from build123d import *

# Parameters (mm, degrees)
BOSS_EXTRUDE1_DEPTH = 4
FILLET1_R           = 3
SKETCH3_R           = 2.6
CUT_EXTRUDE1_DEPTH  = 4
SKETCH4_R           = 1.5
CUT_EXTRUDE2_DEPTH  = 4
SKETCH5_W           = 15
SKETCH5_H           = 20
BOSS_EXTRUDE2_DEPTH = 4
BOSS_EXTRUDE3_DEPTH = 4
SKETCH7_R           = 1.5
CUT_EXTRUDE3_DEPTH  = 4
BOSS_EXTRUDE4_DEPTH = 4
SKETCH10_R          = 11.5
CUT_EXTRUDE4_DEPTH  = 4
SKETCH14_R          = 1.5
CUT_EXTRUDE5_DEPTH  = 4
FILLET2_R           = 3
SKETCH17_W          = 41.796836064
SKETCH17_H          = 42.2
CUT_EXTRUDE6_DEPTH  = 10
FILLET3_R           = 3


with BuildPart() as part:
    # Sketch1 → Boss-Extrude1 (new body)
    with BuildSketch(Plane.XY):
        Polygon((39, 10), (39, 30), (-1, 30), (-9, 10), (-39, 10), (-39, -10), (-9, -10), (-1, -30), (39, -30), (39, -10), align=None)
    extrude(amount=BOSS_EXTRUDE1_DEPTH)

    # Fillet1
    fillet1_edges = [part.edges().sort_by_distance(p)[0] for p in [
        (39, -30, 2),
        (-1, -30, 2),
        (-9, -10, 2),
        (-39, -10, 2),
        (-39, 10, 2),
        (-9, 10, 2),
        (-1, 30, 2),
        (39, 30, 2),
    ]]
    fillet(fillet1_edges, radius=FILLET1_R)

    # Sketch3 → Cut-Extrude1 (cut)
    with BuildSketch(Plane.XY.offset(4)):
        with Locations((33, 20)):
            Circle(SKETCH3_R)
        with Locations((1.6, 20)):
            Circle(SKETCH3_R)
        with Locations((33, -20)):
            Circle(SKETCH3_R)
        with Locations((1.6, -20)):
            Circle(SKETCH3_R)
        with Locations((1.6, 0)):
            Circle(SKETCH3_R)
    extrude(amount=-CUT_EXTRUDE1_DEPTH, mode=Mode.SUBTRACT)

    # Sketch4 → Cut-Extrude2 (cut)
    with BuildSketch(Plane.XY.offset(4)):
        with Locations((-32, 0)):
            Circle(SKETCH4_R)
        with Locations((-25, 0)):
            Circle(SKETCH4_R)
        with Locations((-18, 0)):
            Circle(SKETCH4_R)
        with Locations((-11, 0)):
            Circle(SKETCH4_R)
        with Locations((32, 0)):
            Circle(SKETCH4_R)
        with Locations((25, 0)):
            Circle(SKETCH4_R)
        with Locations((18, 0)):
            Circle(SKETCH4_R)
    extrude(amount=-CUT_EXTRUDE2_DEPTH, mode=Mode.SUBTRACT)

    # Sketch5 → Boss-Extrude2 (add)
    with BuildSketch(Plane.XY.offset(4)):
        with Locations((46.5, 0)):
            Rectangle(SKETCH5_W, SKETCH5_H)
    extrude(amount=-BOSS_EXTRUDE2_DEPTH)

    # Sketch6 → Boss-Extrude3 (add)
    with BuildSketch(Plane.XY.offset(4)):
        Polygon((39, 10), (54, 10), (39, 27), align=None)
        Polygon((54, -10), (39, -10), (39, -27), align=None)
    extrude(amount=-BOSS_EXTRUDE3_DEPTH)

    # Sketch7 → Cut-Extrude3 (cut)
    with BuildSketch(Plane.XY.offset(4)):
        with Locations((46.5, 0)):
            Circle(SKETCH7_R)
    extrude(amount=-CUT_EXTRUDE3_DEPTH, mode=Mode.SUBTRACT)

    # Sketch8 → Boss-Extrude4 (add)
    with BuildSketch(Plane.XY.offset(4)):
        Polygon((54, -10), (54, -21.1), (96.2, -21.1), (96.2, 21.1), (54, 21.1), (54, 10), align=None)
        Polygon((44.205882353, 21.1), (54, 10), (54, 21.1), align=None)
        Polygon((44.205882353, -21.1), (54, -21.1), (54, -10), align=None)
    extrude(amount=-BOSS_EXTRUDE4_DEPTH)

    # Sketch10 → Cut-Extrude4 (cut)
    with BuildSketch(Plane.XY.offset(4)):
        with Locations((74.8, 0)):
            Circle(SKETCH10_R)
    extrude(amount=-CUT_EXTRUDE4_DEPTH, mode=Mode.SUBTRACT)

    # Sketch14 → Cut-Extrude5 (cut)
    with BuildSketch(Plane.XY.offset(4)):
        with Locations((90.674547238, 15.874547238)):
            Circle(SKETCH14_R)
        with Locations((58.925452762, -15.874547238)):
            Circle(SKETCH14_R)
        with Locations((58.925452762, 15.874547238)):
            Circle(SKETCH14_R)
        with Locations((90.674547238, -15.874547238)):
            Circle(SKETCH14_R)
    extrude(amount=-CUT_EXTRUDE5_DEPTH, mode=Mode.SUBTRACT)

    # Fillet2
    fillet2_edges = [part.edges().sort_by_distance(p)[0] for p in [
        (96.2, -21.1, 2),
        (44.205882353, -21.1, 2),
        (44.205882353, 21.1, 2),
        (96.2, 21.1, 2),
        (39, 27, 2),
    ]]
    fillet(fillet2_edges, radius=FILLET2_R)

    # Sketch17 → Cut-Extrude6 (cut)
    with BuildSketch(Plane.XY.offset(4)):
        with Locations((75.301581968, 0)):
            Rectangle(SKETCH17_W, SKETCH17_H)
    extrude(amount=-CUT_EXTRUDE6_DEPTH, mode=Mode.SUBTRACT)

    # Fillet3
    fillet3_edges = [part.edges().sort_by_distance(p)[0] for p in [
        (54.403163936, -21.1, 2),
        (54.403163936, 21.1, 2),
    ]]
    fillet(fillet3_edges, radius=FILLET3_R)


solid = part.part
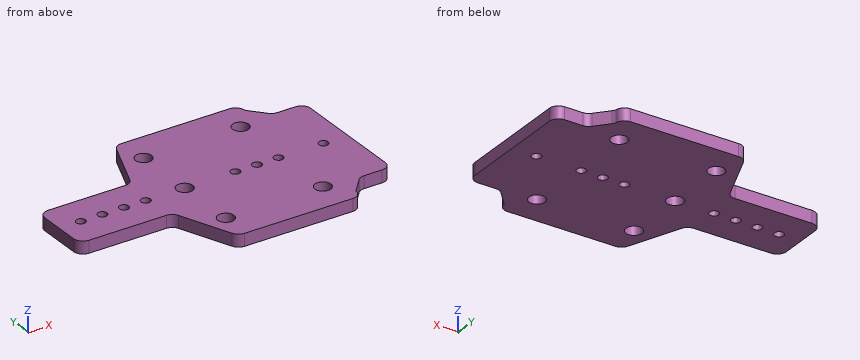
Design review of the part built by this model. Coordinates are the model's own, in mm. Coordinates: 2 decimals unless noted, no trailing zeros. Order: outer loops, then holes, each group sorted by start corner. A loop starts at its lowest first (then second) coordinate and runs counter-clockwise, first axis right, second up.
Item 1: For pin 1 Ø2.5 at (x, y) = (46.5, 0) entering from -Z; pin 2 Ø1.5 at (y, z) = (-12.5, 1) entering from -X; pin 3 Ø2 at (x, z) = (49, 1.5) entering from +Y; pin 4 Ø2 at (x, z) = (-19.5, 3) entering from +Y, all flat-tipped, find the tip position at first contact; note any pin that passes through.
Item 2: For line 1 (Y direction, x = 1.6, z = 1.3); line 2 (Y direction, x = 33, z = 0.9); line 3 (X direction, y = 19.5, z = 2.15), list the stretches that pass through material, from the lowest coordinate up.
Item 3: Take a section at C-C, the plane x = 46.5. Write out the cut boundary in (y, z).
Item 4: Take a section at B-B, the plane y = 0. Count the separate pieces of the cut face and the enclosed holes in it, then the cut area to 3 significant figures.
Item 5: Take a section at A-A, the plane x = 18. Write out the cut boundary in (y, z), then the cut area to 3 significant figures.
The answers:
1. pin 1: passes through
1. pin 2: stops at x = -8.3
1. pin 3: stops at y = 21.1
1. pin 4: stops at y = 10
2. line 1: y = -30 to -22.6, -17.4 to -2.6, 2.6 to 17.4, 22.6 to 30
2. line 2: y = -30 to -22.6, -17.4 to -1.12, 1.12 to 17.4, 22.6 to 30
2. line 3: x = -5.2 to -0.95, 4.15 to 30.45, 35.55 to 54.06
3. outline: (-21.1, 0) - (-1.5, 0) - (-1.5, 4) - (-21.1, 4) - close; (1.5, 0) - (21.1, 0) - (21.1, 4) - (1.5, 4) - close
4. separate pieces: 10
4. enclosed holes: 0
4. area: 257 mm2
5. outline: (-30, 0) - (-1.5, 0) - (-1.5, 4) - (-30, 4) - close; (1.5, 0) - (30, 0) - (30, 4) - (1.5, 4) - close
5. area: 228 mm2
